from build123d import *

# Parameters (mm, degrees)
F0_R     = 8.535
F0_R_2   = 4.725
F1_DEPTH = 2.125
F3_R     = 3.75
F3_R_2   = 2
F4_DEPTH = 12.7
F5_R     = 2.0625
F6_DEPTH = 10.16


with BuildPart() as f1:
    # F0 (on Top) → F1 (new body, symmetric)
    with BuildSketch(Plane.XY):
        Circle(F0_R)
        Circle(F0_R_2, mode=Mode.SUBTRACT)
    extrude(amount=F1_DEPTH, both=True)

    # F3 (on offset) → F4 (join)
    with BuildSketch(Plane.XZ.offset(6.53)):
        Circle(F3_R)
        Circle(F3_R_2, mode=Mode.SUBTRACT)
        Circle(F3_R_2)
    extrude(amount=F4_DEPTH)

    # F5 (on face) → F6 (cut)
    with BuildSketch(Plane.XZ.offset(19.23)):
        Circle(F5_R)
    extrude(amount=-F6_DEPTH, mode=Mode.SUBTRACT)


solid = f1.part
Read the model definition and answer for the solid it produces. Units are mm, in the model's axes. A direction names the side the tool comes from. Coordinates: 2 decimals unless noted, no trailing zeros. Loops run counter-clockwise (first coordinate to the right, second up) from the corner with the lowest first, then second, coordinate; pieces in that order, holes last. Notation, with made-up numbers: (-19, -30) -> (19, -30) arc R16 ccw to (19, 1) -> close; hole circle Ø2 at (56, -32). An arc over 180 degrees is marked (long way). Write item = value, one per line. Start each with the question number.
1) The part is cut by section C-C, the plane z = -1. Determine the outline of the cut face in (x, y) (3 decimals).
2) The part is cut by section D-D, the plane y = 3.75. Determine the outline of the cut face in (x, z) (3 decimals), plus the area to 3 significant figures.
3) The mould has two halves that part along Y. Classify faces 1 (the face through (4.507, 1.419, -0.03)), 2 (the face through (4, 4, -2.125)), 3 (the face through (0, -6.53, 3)): pulls with the +Y half, pulls with the -Y half, needs draft (parallel to the pull), parting line crosses it, or undercut.
4) Find the intervals of material crossed by L1, parallel to Y at x = 0, z = -0.6 (3 decimals); L2, parallel to Z at x = 0, y = -12.5; L3, parallel to Z at x = -4.5, y = 6.25 (3 decimals), in increasing order. Write a range as from..to.
5) The part is cut by section A-A, the plane y = 0. Determine the outline of the cut face in (x, z) (3 decimals), plus the area to 3 significant figures.
6) For faces 4 (the face through (0, -6.53, -3)), 5 (the face through (2, -19.23, -2)), 6 (the face through (0, -9.07, 0)), determine the directions among +Z, -Z, +X, -X, +Y, -Y from which every point of the face is accessible in a straight line to the end or side of a thin tool.
7) Given P1, Ø4, axis at x = 6.5, y = -5.5, coming from the +Z side (3 decimals); P2, Ø1, axis at x = 4.5, z = 0.5, coming from the +Y side; P3, Ø1.5, axis at x = -6, z = -2, coming from the +Y side; P4, Ø7.5, axis at x = 0, y = 0, coming from the +Z side, each flat-ended and moving along its own axis, determine where each tip first touches the part or whether it passes through.
Result:
q1.outline = (-3.614, -19.23) -> (-1.804, -19.23) -> (-1.804, -9.07) -> (1.804, -9.07) -> (1.804, -19.23) -> (3.614, -19.23) -> (3.614, -7.732) arc R8.535 ccw (long way) to (-3.614, -7.732) -> close; hole circle Ø9.45 at (0, 0)
q2.outline = (-7.667, -2.125) -> (-2.875, -2.125) -> (-2.875, 2.125) -> (-7.667, 2.125) -> close; (2.875, -2.125) -> (7.667, -2.125) -> (7.667, 2.125) -> (2.875, 2.125) -> close
q2.area = 40.7 mm²
q3.face_1 = undercut
q3.face_2 = needs draft
q3.face_3 = pulls with the +Y half
q4.L1 = -9.07..-4.725, 4.725..8.535
q4.L2 = -3.75..-2.06, 2.06..3.75
q4.L3 = -2.125..2.125
q5.outline = (-8.535, -2.125) -> (-4.725, -2.125) -> (-4.725, 2.125) -> (-8.535, 2.125) -> close; (4.725, -2.125) -> (8.535, -2.125) -> (8.535, 2.125) -> (4.725, 2.125) -> close
q5.area = 32.4 mm²
q6.face_4 = -Z, +X, -X, +Y
q6.face_5 = +Z, -Z, +X, -X, -Y
q6.face_6 = -Y
q7.P1 = 2.125
q7.P2 = 7.54
q7.P3 = 6.73
q7.P4 = through
